```python
from build123d import *

# Parameters (mm, degrees)
BOSS_EXTRUDE2_DEPTH     = 30
SKETCH5_R               = 11
CUT_EXTRUDE1_DEPTH      = 7
SKETCH6_R               = 5
CUT_EXTRUDE2_DEPTH      = 40
CUT_EXTRUDE3_START      = -7
SKETCH7_R               = 11
CUT_EXTRUDE3_DEPTH      = 7
SKETCH8_W               = 40.5
SKETCH8_H               = 20.5
CUT_EXTRUDE4_DEPTH      = 45
SKETCH9_W               = 15
SKETCH9_H               = 50
CUT_EXTRUDE5_DEPTH      = 45
CUT_EXTRUDE6_DEPTH      = 45
CUT_EXTRUDE6_DEPTH_BACK = 45
SKETCH10_R              = 2
CUT_EXTRUDE7_DEPTH      = 50
CUT_EXTRUDE7_DEPTH_BACK = 45
SKETCH11_R              = 2
FILLET1_R               = 1
SKETCH13_R              = 2
SKETCH13_R_2            = 1.5
BOSS_EXTRUDE3_DEPTH     = 4.75
SKETCH14_R              = 2.5
CUT_EXTRUDE8_DEPTH      = 2.2


with BuildPart() as part:
    # Sketch1 → Revolve2 (revolve)
    with BuildSketch(Plane.XY, mode=Mode.PRIVATE) as revolve2_sk:
        with BuildLine():
            Line((0, 2.25), (0, 5))
            Line((0, 5), (-20, 5))
            Line((-20, 5), (-20, -5))
            Line((-20, -5), (0, -5))
            Line((0, -5), (0, -2.25))
            ThreePointArc((0, -2.25), (-2.25, 0), (0, 2.25))
        make_face()
    revolve(revolve2_sk.sketch.rotate(Axis((-20, 5, 0), (0, -1, 0)), 90), axis=Axis((-20, 5, 0), (0, -1, 0)))

    # Sketch4 → Boss-Extrude2 (add)
    with BuildSketch(Plane(origin=(0, 5, 0), x_dir=(1, 0, 0), z_dir=(0, 1, 0))):
        with BuildLine():
            Line((-7.390479787, 25), (50, 25))
            Line((50, 25), (50, -25))
            Line((50, -25), (-7.390479787, -25))
            ThreePointArc((-7.390479787, -25), (-48, 0), (-7.390479787, 25))
        make_face()
    extrude(amount=BOSS_EXTRUDE2_DEPTH)

    # Sketch5 → Cut-Extrude1 (cut)
    with BuildSketch(Plane.XZ.offset(5)):
        with Locations(Location((-20, 0, 0), (0, 0, 270))):
            Circle(SKETCH5_R)
    extrude(amount=-CUT_EXTRUDE1_DEPTH, mode=Mode.SUBTRACT)

    # Sketch6 → Cut-Extrude2 (cut)
    with BuildSketch(Plane.XZ.offset(-2)):
        with Locations(Location((-20, 0, 0), (0, 0, 270))):
            Circle(SKETCH6_R)
    extrude(amount=-CUT_EXTRUDE2_DEPTH, mode=Mode.SUBTRACT)

    # Sketch7 → Cut-Extrude3 (cut)
    with BuildSketch(Plane(origin=(0, 35, 0), x_dir=(1, 0, 0), z_dir=(0, 1, 0)).offset(CUT_EXTRUDE3_START)):
        with Locations(Location((-20, 0, 0), (0, 0, 90))):
            Circle(SKETCH7_R)
    extrude(amount=CUT_EXTRUDE3_DEPTH, mode=Mode.SUBTRACT)

    # Sketch8 → Cut-Extrude4 (cut)
    with BuildSketch(Plane(origin=(50, 0, 0), x_dir=(0, 0, -1), z_dir=(1, 0, 0))):
        with Locations((0, 20)):
            Rectangle(SKETCH8_W, SKETCH8_H)
    extrude(amount=-CUT_EXTRUDE4_DEPTH, mode=Mode.SUBTRACT)

    # Sketch9 → Cut-Extrude5 (cut)
    with BuildSketch(Plane(origin=(0, 35, 0), x_dir=(1, 0, 0), z_dir=(0, 1, 0))):
        with Locations((42.5, 0)):
            Rectangle(SKETCH9_W, SKETCH9_H)
    extrude(amount=-CUT_EXTRUDE5_DEPTH, mode=Mode.SUBTRACT)

    # Sketch10 → Cut-Extrude6 (cut, two sides: drawn at the far end of the back side and taken through both)
    with BuildSketch(Plane.XZ.offset(-30.25).offset(-CUT_EXTRUDE6_DEPTH_BACK)):
        with Locations(Location((25, 9.75, 0), (0, 0, 90))):
            Circle(SKETCH10_R)
        with Locations(Location((25, -10.25, 0), (0, 0, 90))):
            Circle(SKETCH10_R)
    extrude(amount=CUT_EXTRUDE6_DEPTH + CUT_EXTRUDE6_DEPTH_BACK, mode=Mode.SUBTRACT)

    # Sketch11 → Cut-Extrude7 (cut, two sides: drawn at the far end of the back side and taken through both)
    with BuildSketch(Plane.XY.offset(-20.25).offset(-CUT_EXTRUDE7_DEPTH_BACK)):
        with Locations(Location((25, 20, 0), (0, 0, 90))):
            Circle(SKETCH11_R)
    extrude(amount=CUT_EXTRUDE7_DEPTH + CUT_EXTRUDE7_DEPTH_BACK, mode=Mode.SUBTRACT)

    # Fillet1
    fillet1_edges = [part.edges().sort_by_distance(p)[0] for p in [
        (-48, 5, 0),
        (13.804760106, 5, 25),
        (-48, 35, 0),
        (13.804760106, 35, 25),
        (13.804760106, 35, -25),
        (13.804760106, 5, -25),
    ]]
    fillet(fillet1_edges, radius=FILLET1_R)

    # Sketch13 → Boss-Extrude3 (add)
    # profile 1 of 2: a face of its own
    with BuildSketch(Plane.XZ.offset(-5)):
        with Locations(Location((25, 9.75, 0), (0, 0, 90))):
            Circle(SKETCH13_R)
        with Locations(Location((25, 9.75, 0), (0, 0, 270))):
            Circle(SKETCH13_R_2, mode=Mode.SUBTRACT)
    # profile 2 of 2: a face of its own
    with BuildSketch(Plane.XZ.offset(-5)):
        with Locations(Location((25, -10.25, 0), (0, 0, 90))):
            Circle(SKETCH13_R)
        with Locations(Location((25, -10.25, 0), (0, 0, 270))):
            Circle(SKETCH13_R_2, mode=Mode.SUBTRACT)
    extrude(amount=-BOSS_EXTRUDE3_DEPTH)

    # Sketch14 → Cut-Extrude8 (cut)
    with BuildSketch(Plane.XZ.offset(-5)):
        with Locations(Location((25, 9.75, 0), (0, 0, 270))):
            Circle(SKETCH14_R)
        with Locations(Location((25, -10.25, 0), (0, 0, 270))):
            Circle(SKETCH14_R)
    extrude(amount=-CUT_EXTRUDE8_DEPTH, mode=Mode.SUBTRACT)


solid = part.part
```
The listing builds one solid part. Answer for the finished solid, in the listing's coordinates (mm). A direction names the side the tool comes from. Give positions to 0.01 mm unless a question says otherwise; leave off trailing zeros. Order: outer loops, then holes, each group sorted by start corner. A loop starts at its lowest first (then second) coordinate and runs counter-clockwise, first axis right, second up. Notation, with made-up numbers: (79.5, -31) - (89.5, -31) arc R18 cw to (89.5, 4) - close; hole circle Ø1 at (83.5, 36). An arc over 180 degrees is marked (long way). Use one line per item in the form item = value. Start each with the question number.
(1) A cutting plane is placed at A-A, the plane y = 20. Write down the section's boundary in (x, z), then the cut area to 3 significant figures.
(2) A cutting plane is placed at D-D, the plane y = 12.5. Write down the section's boundary in (x, z), then the cut area to 3 significant figures.
(3) The mould has two halves that part along Y. Classify faces 4 (the cylindrical face through (-47.99, 19.8, 0.8)), 5 (the flat face through (20, 9.75, 0)), 6 (the flat face through (-5, 35, 0)): released by +Y, released by -Y, zero draft, split by the parting line, or undercut.
(4) For faces 1 (the flat face through (20, 20, 20.25)), 2 (the cylindrical face through (-9.26, 31.45, 2.38)), 3 (the flat face through (25, 7.2, -12)), determine the directions among +Z, -Z, +X, -X, +Y, -Y from which every point of the face is accessible in a straight line to the end or side of a thin tool.
(5) A cutting plane is placed at C-C, the plane x = 10. Write down the section's boundary in (y, z).
(6) Consider line 1 (X direction, y = 19, z = 0); line 2 (Y direction, x = 25.5, z = -12.5); line 3 (Z direction, x = 31.5, y = 25). Determine where each line is inside the solid, lowest interval first. Write a range as from..to.
(7) Flat-ended cylindrical pins translate along their axes: pin 1 Ø8 at (x, y) = (-38, 7.5) entering from +Z; pin 2 Ø2.5 at (x, z) = (25, -10.25) entering from +Y; pin 3 Ø4.5 at (x, z) = (25, 9.75) entering from -Y; pin 4 Ø20 at (x, z) = (-20, 0) entering from +Y. Find the tip coordinate at first contact, or state that the pin passes through.
Ans:
q1.outline = (-7.39, -25) - (23, -25) - (23, -20.25) - (5, -20.25) - (5, 20.25) - (23, 20.25) - (23, 25) - (-7.39, 25) arc R28 ccw (long way) to start; (27, -25) - (35, -25) - (35, -20.25) - (27, -20.25) - close; (27, 20.25) - (35, 20.25) - (35, 25) - (27, 25) - close; hole circle Ø10 at (-20, 0)
q1.area = 2,700 mm^2
q2.outline = (-7.39, -25) - (35, -25) - (35, -20.25) - (5, -20.25) - (5, 20.25) - (35, 20.25) - (35, 25) - (-7.39, 25) arc R28 ccw (long way) to start; hole circle Ø10 at (-20, 0)
q2.area = 2,740 mm^2
q3.face_4 = zero draft
q3.face_5 = undercut
q3.face_6 = released by +Y
q4.face_1 = +X
q4.face_2 = +Y
q4.face_3 = -Y
q5.outline = (5, -24) arc R1 ccw to (6, -25) - (34, -25) arc R1 ccw to (35, -24) - (35, 24) arc R1 ccw to (34, 25) - (6, 25) arc R1 ccw to (5, 24) - close; hole (9.75, -20.25) - (30.25, -20.25) - (30.25, 20.25) - (9.75, 20.25) - close
q6.line_1 = -48..-25, -15..5
q6.line_2 = 7.2..9.75, 30.25..35
q6.line_3 = -25..-20.25, 20.25..25
q7.pin_1 = 24.25
q7.pin_2 = through
q7.pin_3 = 7.2
q7.pin_4 = 28
